Could you check a few things on this drawing? It's one solid part, dimensions in mm from its lowest x, y, z. Coordinates: 2 decimals unless noted, no trailing zeros. Order: outer loops, then holes, each group sorted by start corner. A loop starts at its lowest first (then second) coordinate and runs counter-clockwise, first axis right, second up.
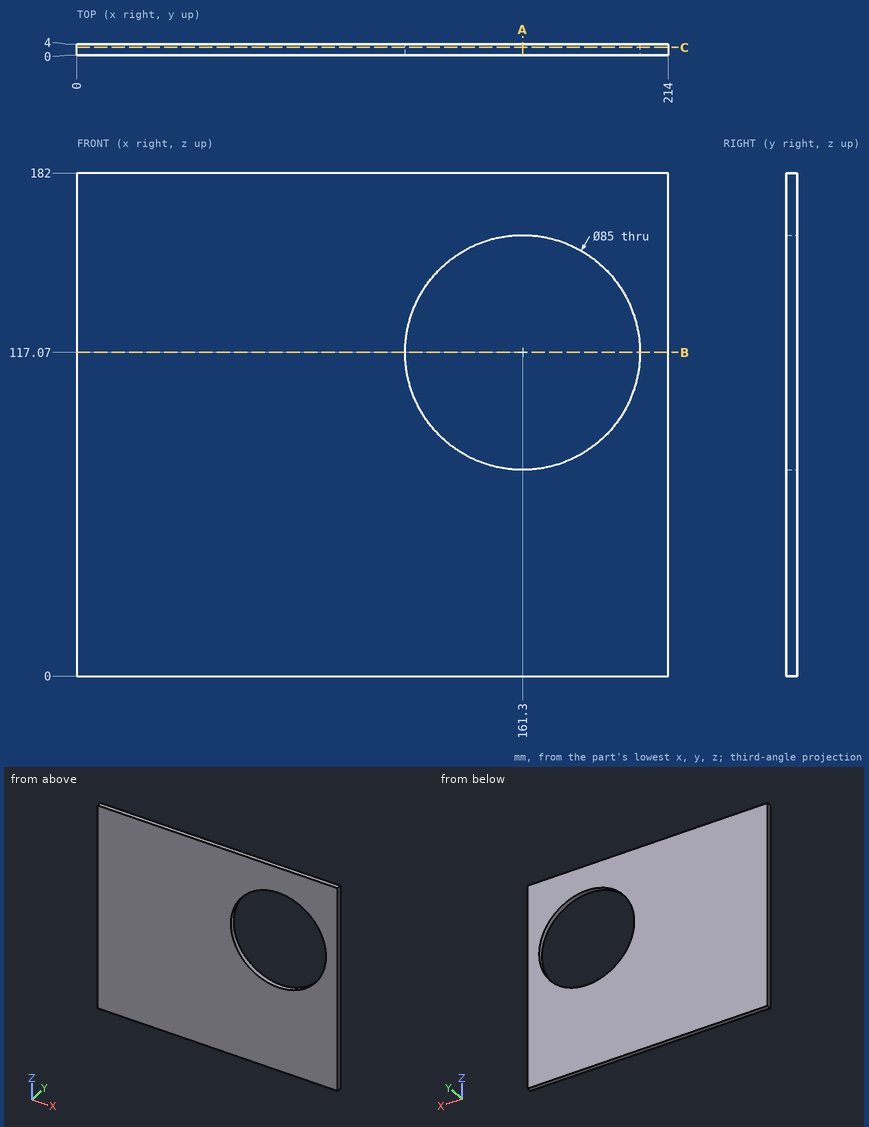
Item 1: Suppose I cut it at A-A (x = 161.3). List the corners of the cut face in (y, z) for me, and give its area (3 significant figures).
Item 2: For pin 1 Ø12 at (x, z) = (125, 126) entering from +Y, with a flat end and sliding along its axis, tell me the tip position at first contact or that it passes through.
Item 3: Suppose I cut it at C-C (y = 2.75). List the corners of the cut face in (x, z) for me, and give its area (3 significant figures).
Item 4: Suppose I cut it at B-B (z = 117.07). List the corners of the cut face in (x, y) for me, and give its area (3 significant figures).
Item 5: I need wall thicknesses on line 1 (Z direction, x = 161.3, y = 1.45); line 2 (X direction, y = 1.3, z = 117.07); line 3 (X direction, y = 2.15, z = 138). Which ranges of each line are inside material? Lowest first, please.
Geometry results:
1. outline: (0, 0) - (4, 0) - (4, 74.57) - (0, 74.57) - close; (0, 159.57) - (4, 159.57) - (4, 182) - (0, 182) - close
1. area: 388 mm2
2. pin 1: stops at y = 4
3. outline: (0, 0) - (214, 0) - (214, 182) - (0, 182) - close; hole circle Ø85 at (161.3, 117.07)
3. area: 33,300 mm2
4. outline: (0, 0) - (118.8, 0) - (118.8, 4) - (0, 4) - close; (203.8, 0) - (214, 0) - (214, 4) - (203.8, 4) - close
4. area: 516 mm2
5. line 1: z = 0 to 74.57, 159.57 to 182
5. line 2: x = 0 to 118.8, 203.8 to 214
5. line 3: x = 0 to 124.31, 198.29 to 214
